Input: part model. Units: mm. Frame: model coordinates. Coordinates: 2 decimals unless noted, no trailing zeros. Write each loop counter-clockwise with the first axis right and the second up, starting at its lowest first coordinate (ties: lowest second). Pieces come first, ordered by that corner, then holes. Notation, with made-up numbers: M -8,31 L 4,31 A13 ccw 4,39 Z; hole C -20,-26 d7. An arc over 180 degrees is marked long. Write each question's results on one line, items separated by ' | '. Start each with the question number.
1. Pull-direction query (Y, two-part tool) for faces 1 (the flat face through (9, 1, 0)), 2 (the cylindrical face through (-1.08, -4.88, 2.54)), 3 (the cylindrical face through (-5.598, 42.634, 2.493)); classes: +Y half, -Y half, draft (parallel to the pull), parting line (faces both ways), or undercut.
2. Ray query, probe 1 along Y at (x, z) = (0, 1.85); probe 2 along X at (y, z) = (25.5, 0.4); probe 3 along Y at (x, z) = (0, 3.8). Return the intervals inside material, ascending.
3. Section query A-A, the plane x = 0. Output: boundary loops of the cut face in (y, z).
4. First-contact query: pin 1 (1 mm diameter, centred on x = -12, z = 4, fed in from +Y); pin 2 (1.5 mm diameter, centred on y = 24.5, z = 1.5, fed in from -X); pin 3 (1 mm diameter, centred on x = -4.5, z = 4, fed in from +Y). Flat tips, straight axial feed; report the tip coordinate or a pass-through.
```python
from build123d import *

# Parameters (mm, degrees)
F0_R     = 43
F1_DEPTH = 5
F2_R     = 5
F3_DEPTH = 5.001
F4_R     = 2


with BuildPart() as f1:
    # F0 (on Top) → F1 (new body)
    with BuildSketch(Plane.XY):
        Circle(F0_R)
    extrude(amount=F1_DEPTH)

    # F2 (on face) → F3 (cut, through all)
    with BuildSketch(Plane.XY.offset(5)):
        Circle(F2_R)
    extrude(amount=-F3_DEPTH, mode=Mode.SUBTRACT)

    # F4
    f4_edges = [f1.edges().sort_by_distance(p)[0] for p in [
        (-43, 0, 0),
        (-43, 0, 5),
    ]]
    fillet(f4_edges, radius=F4_R)


solid = f1.part
```
Answer:
1) face 1: draft | face 2: undercut | face 3: parting line
2) probe 1: -42.99 to -5, 5 to 42.99 | probe 2: -33.62 to 33.62 | probe 3: -42.83 to -5, 5 to 42.83
3) outline: M -43,2 A2 ccw -41,0 L -5,0 L -5,5 L -41,5 A2 ccw -43,3 Z; M 5,0 L 41,0 A2 ccw 43,2 L 43,3 A2 ccw 41,5 L 5,5 Z
4) pin 1: y = 41.28 | pin 2: x = -35.8 | pin 3: y = 42.71
